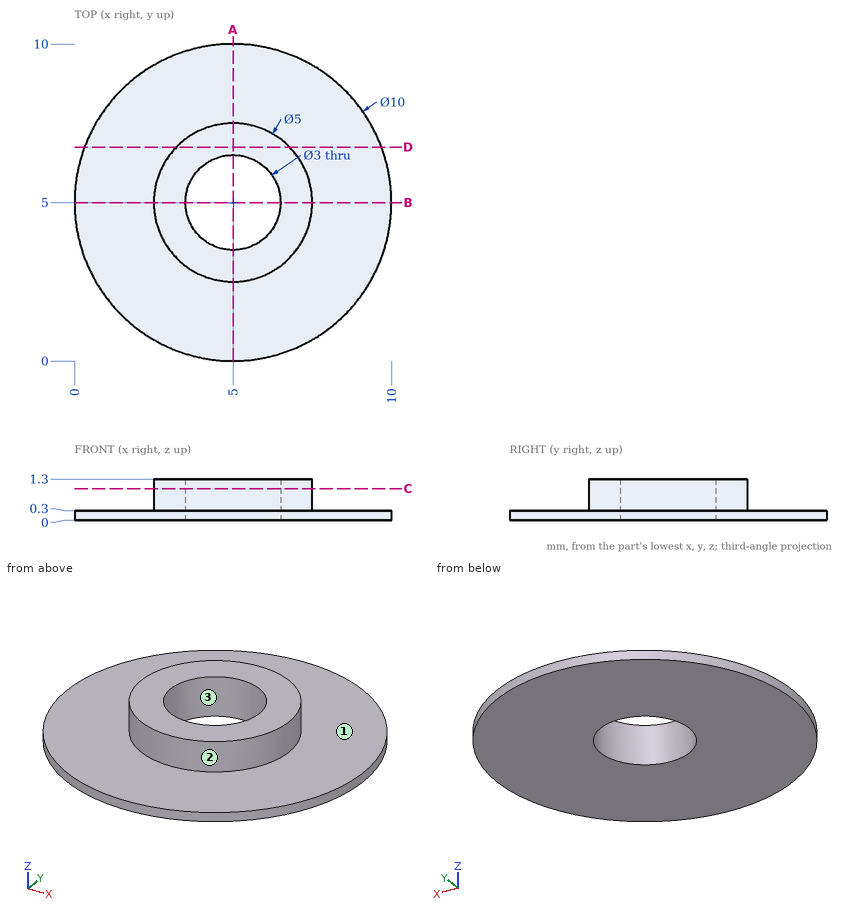
Part print with two shaded views. Sizes in mm from the minimum x, y, z corner. Round coordinates to 2 decimals unless told otherwise and drop trailing zeros. Order: outer loops, then holes, each group sorted by start corner. A loop starts at its lowest first (then second) coordinate and runs counter-clockwise, first axis right, second up.
(1) Band-saw the part on D-D (y = 6.75). List the corners of the cut face in (x, z), then the cut area to 3 significant figures.
(2) Drill centre lines: line 1 (Y direction, x = 5, z = 0.85); line 2 (Z direction, x = 3.25, y = 8.25); line 3 (X direction, y = 3, z = 0.9). Where is each one in solid material? Low to high.
(3) Band-saw the part on A-A (x = 5). List the corners of the cut face in (y, z), then the cut area to 3 significant figures.
(4) Band-saw the part on C-C (z = 1). List the corners of the cut face in (x, y), then the cut area to 3 significant figures.
(5) Pin check, flat tips, straight feed: pin 1 (2 mm diameter, centred on x = 3.5, y = 6, fed in from -Z); pin 2 (4 mm diameter, centred on x = 2, y = 1, fed in from +Z). Stop position of each tip, or through.
(6) Pull direction X, two halves, no side cores. Call the marked faces 1, 2 and 3: released by +X, released by -X, zero draft, split by the parting line, or undercut.
Verdict:
1. outline: (0.32, 0) - (9.68, 0) - (9.68, 0.3) - (6.79, 0.3) - (6.79, 1.3) - (3.21, 1.3) - (3.21, 0.3) - (0.32, 0.3) - close
1. area: 6.38 mm2
2. line 1: y = 2.5 to 3.5, 6.5 to 7.5
2. line 2: z = 0 to 0.3
2. line 3: x = 3.5 to 6.5
3. outline: (0, 0) - (3.5, 0) - (3.5, 1.3) - (2.5, 1.3) - (2.5, 0.3) - (0, 0.3) - close; (6.5, 0) - (10, 0) - (10, 0.3) - (7.5, 0.3) - (7.5, 1.3) - (6.5, 1.3) - close
3. area: 4.10 mm2
4. outline: circle Ø5 at (5, 5); hole circle Ø3 at (5, 5)
4. area: 12.6 mm2
5. pin 1: stops at z = 0
5. pin 2: stops at z = 0.3
6. face 1: zero draft
6. face 2: split by the parting line
6. face 3: undercut
